from build123d import *

# Parameters (mm, degrees)
SKETCH004_W     = 43
SKETCH004_H     = 68.9
PAD001_DEPTH    = 1.6
SKETCH005_W     = 18
SKETCH005_H     = 34
PAD002_DEPTH    = 6.3
SKETCH006_W     = 17.1
SKETCH006_H     = 57
PAD003_DEPTH    = 15.5
FILLET_R        = 7
POCKET003_DEPTH = 3.601
SKETCH010_W     = 19
SKETCH010_H     = 19
PAD004_DEPTH    = 13


with BuildPart() as part:
    # Sketch004 → Pad001 (new body)
    with BuildSketch(Plane.XY):
        with Locations((0, -34.45)):
            Rectangle(SKETCH004_W, SKETCH004_H)
    extrude(amount=-PAD001_DEPTH)

    # Sketch005 → Pad002 (join)
    with BuildSketch(Plane.XY):
        with Locations((0, -17)):
            Rectangle(SKETCH005_W, SKETCH005_H)
    extrude(amount=PAD002_DEPTH)

    # Sketch006 → Pad003 (join)
    with BuildSketch(Plane.XY.offset(-3.6)):
        with Locations((-19, -32.2)):
            Rectangle(SKETCH006_W, SKETCH006_H)
    extrude(amount=PAD003_DEPTH)

    # Fillet
    fillet_edges = [part.edges().sort_by_distance(p)[0] for p in [
        (-10.45, -32.2, 11.9),
        (-27.55, -32.2, 11.9),
    ]]
    fillet(fillet_edges, radius=FILLET_R)

    # Sketch009 → Pocket003 (cut, through all)
    with BuildSketch(Plane.XY):
        with BuildLine():
            ThreePointArc((-20.1, -63.1), (-19, -64.2), (-17.9, -63.1))
            Line((-17.9, -63.1), (-17.9, -62.3))
            ThreePointArc((-17.9, -62.3), (-19, -61.2), (-20.1, -62.3))
            Line((-20.1, -62.3), (-20.1, -63.1))
        make_face()
        with BuildLine():
            ThreePointArc((-17.9, -1.3), (-19, -0.2), (-20.1, -1.3))
            Line((-20.1, -1.3), (-20.1, -2.1))
            ThreePointArc((-20.1, -2.1), (-19, -3.2), (-17.9, -2.1))
            Line((-17.9, -2.1), (-17.9, -1.3))
        make_face()
    extrude(amount=-POCKET003_DEPTH, mode=Mode.SUBTRACT)

    # Sketch010 → Pad004 (join)
    with BuildSketch(Plane.XY):
        with Locations((0, -49)):
            Rectangle(SKETCH010_W, SKETCH010_H)
    extrude(amount=PAD004_DEPTH)


solid = part.part
Read the model definition and answer for the solid it produces. Units are mm, in the model's axes. A direction names the side the tool comes from. Give positions to 0.01 mm unless a question says otherwise; leave off trailing zeros. Write each loop counter-clockwise with the first axis right and the second up, starting at its lowest first coordinate (ties: lowest second). Pieces come first, ordered by that corner, then holes. Notation, with made-up numbers: (-4, 44) - (34, 44) arc R24 ccw to (34, 75) - close; hole circle Ø5 at (57, 34). An arc over 180 degrees is marked (long way). Use CSV: the item, a comma, the result in double quotes. Start each with the question number.
Item 1: The mould has two halves that part along X. Classify faces 6 (the flat face through (-21.5, -65, -1)), 7 (the flat face through (-19, -32, 11.9)), 8 (the flat face through (-9.5, -49, 6)), 9 (the cylindrical face through (-12.55, -31.8, 9.9)): pulls with the +X half, pulls with the -X half, needs draft (parallel to the pull), parting line crosses it, or undercut.
Item 2: The part is cut by section A-A, the plane x = -19. Give the vertices of the cut face in (y, z).
Item 3: The part is cut by section D-D, the plane z = 8.25. Give the vertices of the cut face in (x, y).
Item 4: Flat-ended cylindrical pins translate along their axes: P1, Ø1, axis at x = 10.5, y = -38, coming from the +Z side; P2, Ø6.5, axis at x = -4, z = 6, coming from the -Y side; P3, Ø4, axis at y = -48, z = 7.5, coming from the +X side; P4, Ø8, axis at x = 15, z = 10.5, coming from the -Y side. Find the tip coordinate at first contact, or state that the pin passes through.
Item 5: For faces 1 (the flat face through (9.5, -49, 6)), 2 (the flat face through (0, -17, 6.3)), 3 (the flat face through (0, -58.5, 6)), 4 (the cylindrical face through (-19, -61.2, -0.8)), 5 (the flat face through (-21.5, -2, -1)), determine the directions among +Z, -Z, +X, -X, +Y, -Y from which every point of the face is accessible in a straight line to the end or side of a thin tool.
Item 6: The part is cut by section B-B, the plane z = 3.5. Give the vertices of the cut face in (x, y).
Item 7: The part is cut by section C-C, the plane y = -16.5. Give the vertices of the cut face in (x, z), and give its area (3 significant figures).
Item 8: Consider line 1 (X direction, y = -20, z = 1.25); line 2 (Y direction, x = -0.5, z = 2.75); line 3 (Z direction, x = -19, y = -19). Determine where each line is inside the solid, lowest interval first.
Taken from the geometry:
1,face 6,"pulls with the -X half"
1,face 7,"needs draft"
1,face 8,"undercut"
1,face 9,"undercut"
2,outline,"(-68.9, -1.6) - (-64.2, -1.6) - (-64.2, 0) - (-68.9, 0) - close; (-61.2, -1.6) - (-60.7, -1.6) - (-60.7, -3.6) - (-3.7, -3.6) - (-3.7, -1.6) - (-3.2, -1.6) - (-3.2, 0) - (-3.7, 0) - (-3.7, 11.9) - (-60.7, 11.9) - (-60.7, 0) - (-61.2, 0) - close; (-0.2, -1.6) - (0, -1.6) - (0, 0) - (-0.2, 0) - close"
3,outline,"(-26.7, -60.7) - (-11.3, -60.7) - (-11.3, -3.7) - (-26.7, -3.7) - close; (-9.5, -58.5) - (9.5, -58.5) - (9.5, -39.5) - (-9.5, -39.5) - close"
4,P1,"z = 0"
4,P2,"y = -58.5"
4,P3,"x = 9.5"
4,P4,"through"
5,face 1,"+Z, +X, +Y, -Y"
5,face 2,"+Z, +X, +Y"
5,face 3,"+Z, +X, -Y"
5,face 4,"+Z, -Z"
5,face 5,"+Z, -Z, -X, +Y"
6,outline,"(-27.55, -60.7) - (-10.45, -60.7) - (-10.45, -3.7) - (-27.55, -3.7) - close; (-9.5, -58.5) - (9.5, -58.5) - (9.5, -39.5) - (-9.5, -39.5) - close; (-9, -34) - (9, -34) - (9, 0) - (-9, 0) - close"
7,outline,"(-27.55, -3.6) - (-10.45, -3.6) - (-10.45, -1.6) - (21.5, -1.6) - (21.5, 0) - (9, 0) - (9, 6.3) - (-9, 6.3) - (-9, 0) - (-10.45, 0) - (-10.45, 4.9) arc R7 ccw to (-17.45, 11.9) - (-20.55, 11.9) arc R7 ccw to (-27.55, 4.9) - close"
7,area,"409 mm2"
8,line 1,"-27.55 to -10.45, -9 to 9"
8,line 2,"-58.5 to -39.5, -34 to 0"
8,line 3,"-3.6 to 11.9"
